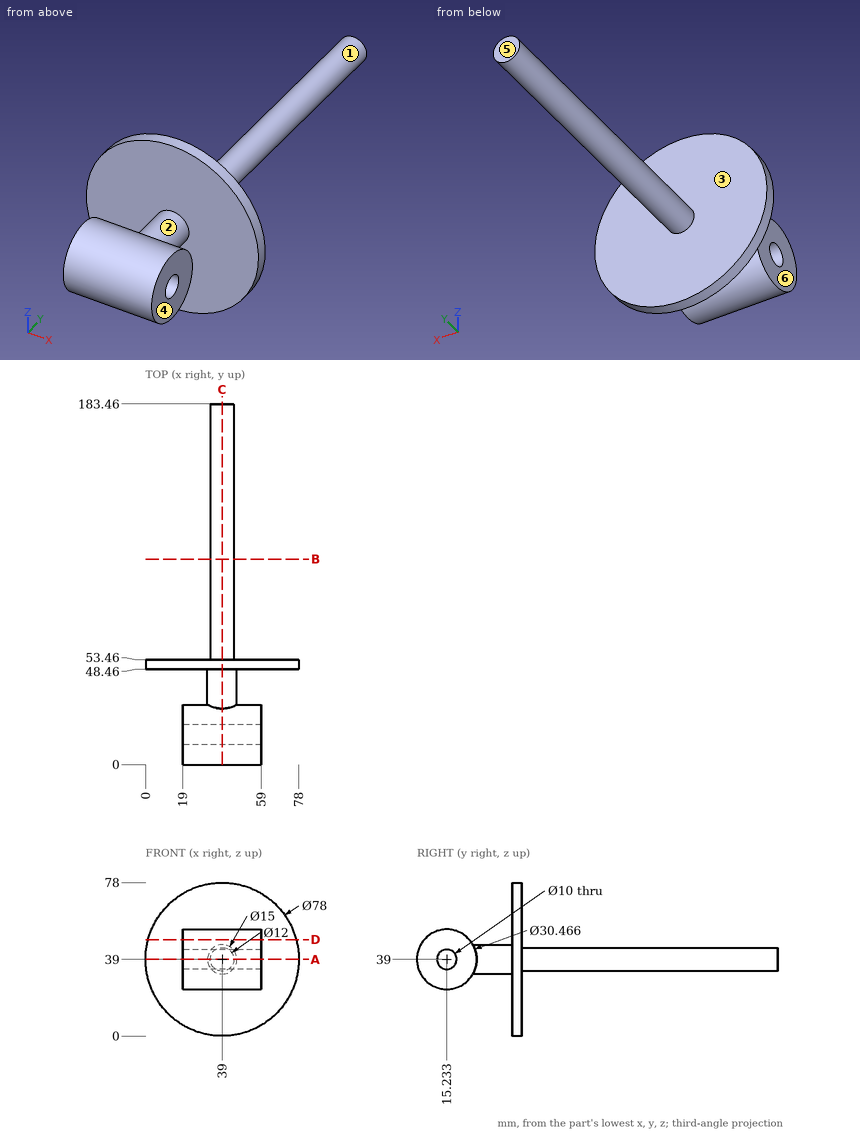
Can you work these out from the drawing? Everything is in mm from the part's minimum corner. A direction names the side the tool comes from. Give positions to 0.01 mm unless a question says otherwise; leave off trailing zeros. Loops run counter-clockwise (first coordinate to the right, second up) from the corner with the lowest first, then second, coordinate; pieces in that order, holes last. Notation, with made-up numbers: (38.25, -26) -> (45.25, -26) arc R19 ccw to (45.25, 11) -> close; hole circle Ø9 at (75, 29). An arc over 180 degrees is marked (long way). Write item = value, one per line.
1) Suppose I cut it at C-C on x = 39. Write out the boundary of the cut face in (y, z), then the cut area to 3 significant figures.
Check result:
outline = (28.49, 31.5) -> (48.46, 31.5) -> (48.46, 0) -> (53.46, 0) -> (53.46, 33) -> (183.46, 33) -> (183.46, 45) -> (53.46, 45) -> (53.46, 78) -> (48.46, 78) -> (48.46, 46.5) -> (28.49, 46.5) arc R15.23 ccw (long way) to start; hole circle Ø10 at (15.23, 39)
area = 2,880 mm2
2) I need wall thicknesses on L1, parallel to Y at x = 38, z = 39; L2, parallel to Y at x = 48.5, z = 39; L3, parallel to Y at x = 63, z = 40.5. Which ranges of each line are inside material? Lowest first, please. Write a range as from..to.
Check result:
L1 = 0..10.23, 20.23..183.46
L2 = 0..10.23, 20.23..30.47, 48.46..53.46
L3 = 48.46..53.46
3) Thinking about a two-plate mould opening in Y: for the marked faces 1, 2 and 3, which applies, released by +Y, released by -Y, zero draft, split by the parting line, or undercut?
Check result:
face_1 = zero draft
face_2 = undercut
face_3 = released by +Y
4) Suppose I cut it at D-D on z = 49. Write out the boundary of the cut face in (x, y) (1 decimal), then the cut area to 3 significant figures.
Check result:
outline = (1.3, 48.5) -> (76.7, 48.5) -> (76.7, 53.5) -> (1.3, 53.5) -> close; (19, 3.7) -> (59, 3.7) -> (59, 26.7) -> (19, 26.7) -> close
area = 1,300 mm2
5) Suppose I cut it at A-A on z = 39. Write out the boundary of the cut face in (x, y).
Check result:
outline = (0, 48.46) -> (31.5, 48.46) -> (31.5, 30.47) -> (19, 30.47) -> (19, 20.23) -> (59, 20.23) -> (59, 30.47) -> (46.5, 30.47) -> (46.5, 48.46) -> (78, 48.46) -> (78, 53.46) -> (45, 53.46) -> (45, 183.46) -> (33, 183.46) -> (33, 53.46) -> (0, 53.46) -> close; (19, 0) -> (59, 0) -> (59, 10.23) -> (19, 10.23) -> close
6) Will these pins go through, and if not, where does the flat tip stop? pin 1 (1.5 mm diameter, centred on y = 50, z = 32.5, fed in from +X); pin 2 (12 mm diameter, centred on x = 32, y = 90.5, fed in from +Z); pin 3 (16 mm diameter, centred on y = 15.23, z = 39, fed in from +X).
Check result:
pin_1 = 77.57
pin_2 = 44.92
pin_3 = 59
7) For the marked faces 4, 5 and 6, which set-ups out of +Z, -Z, +X, -X, +Y, -Y let a thin tool reach every point of the face, with its end or its side?
Check result:
face_4 = +Z, -Z, +X, -Y
face_5 = +Z, -Z, +X, -X, +Y
face_6 = +Z, -Z, -X, -Y
8) Suppose I cut it at B-B on y = 104.5. Write out the boundary of the cut face in (x, z), then the cut area to 3 significant figures.
Check result:
outline = circle Ø12 at (39, 39)
area = 113 mm2
